Check sheet for the drawn part. Datum: minimum x, y, z corner. Units: mm. A direction names the side the tool comes from. Give positions to 0.01 mm unless a question says otherwise; leave off trailing zeros. Order: outer loops, then holes, each group sorted by start corner. A loop starts at its lowest first (then second) coordinate and runs counter-clockwise, first axis right, second up.
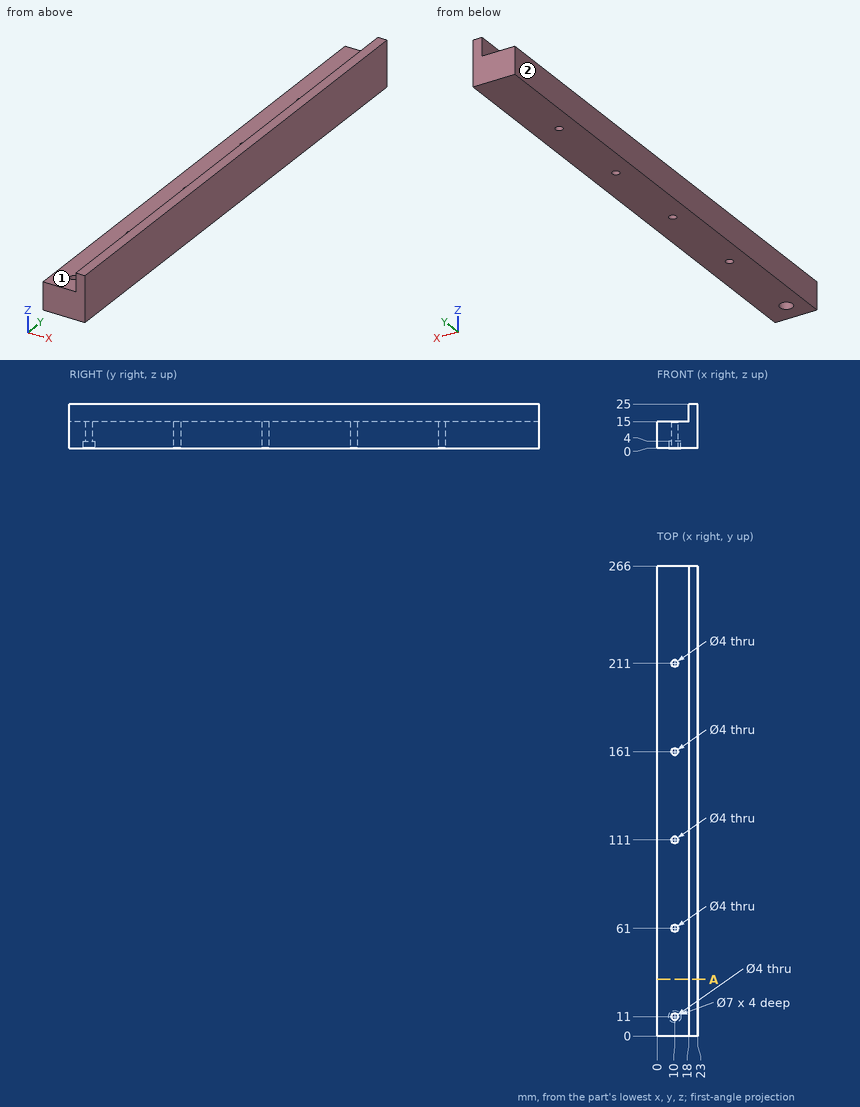
Item 1: Sectioned sample at A-A (y = 32). Enter the section's corners in (x, z), and give its area (3 significant figures).
Reported:
outline: (0, 0) - (23, 0) - (23, 25) - (18, 25) - (18, 15) - (0, 15) - close
area: 395 mm2
Item 2: Gauge pin test, flat ends, axial feed: pin 1 (3 mm diameter, centred on x = 11.5, y = 46.5, fed in from +Z); pin 2 (3.5 mm diameter, centred on x = 10, y = 211, fed in from +Z); pin 3 (5.5 mm diameter, centred on x = 10, y = 11, fed in from -Z). Record the tip position at first contact, or that the pin passes through.
Reported:
pin 1: stops at z = 15
pin 2: passes through
pin 3: stops at z = 4
Item 3: Scan lines: L1, parallel to Y at x = 10, z = 9.5; L2, parallel to X at y = 161, z = 6; L3, parallel to Y at x = 10, z = 0.8. Record each from-to range of solid material in increasing order.
Reported:
L1: y = 0 to 9, 13 to 59, 63 to 109, 113 to 159, 163 to 209, 213 to 266
L2: x = 0 to 8, 12 to 23
L3: y = 0 to 7.5, 14.5 to 59, 63 to 109, 113 to 159, 163 to 209, 213 to 266
Item 4: Set-up check for the marked faces 1 and 2: record each of +Z, -Z, +X, -X, +Y, -Y from which the full face is reachable in a straight line by a thin tool's end or side.
Reported:
face 1: +Z, -X, +Y, -Y
face 2: +Z, -Z, -X, +Y, -Y
